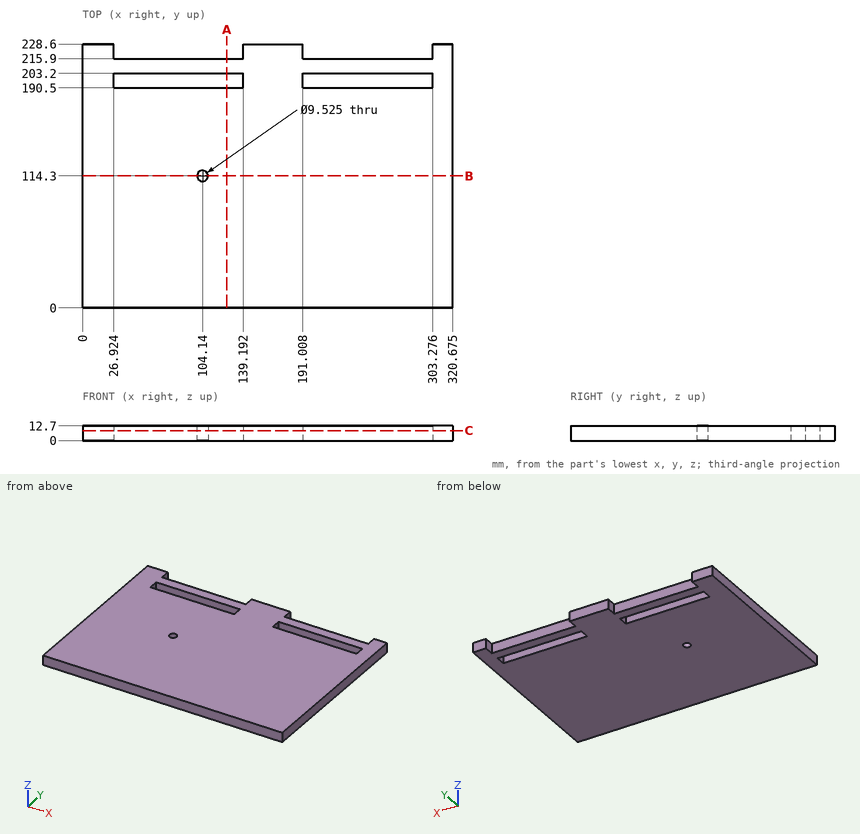
Print and shaded views of the part. All mm, measured from the part's lowest x, y and z. Round coordinates to 2 decimals unless told otherwise and drop trailing zeros. Order: outer loops, then holes, each group sorted by start corner. A loop starts at its lowest first (then second) coordinate and runs counter-clockwise, first axis right, second up.
Q1. Wall check: L1, parallel to X at y = 198, z = 9.75 (3 decimals); L2, parallel to Y at x = 104.14, z = 3.25; L3, parallel to Y at x = 86, z = 11.5. Give the ranges that are in metal, low to high.
Q2. Slice it at B-B (y = 114.3). Write the cut outline in (x, z) (1 decimal).
Q3. Drop a flat-ended pin along its axis: pin 1 (1 mm diameter, centred on x = 260, z = 5, fed in from +Y). Give the stop position or say it passes through.
Q4. Slice it at C-C (z = 8.5). Write the cut outline in (x, y) (1 decimal).
Q5. Slice it at A-A (x = 125). Write the cut outline in (y, z), and give its area (3 significant figures).
Results below:
1. L1: x = 0 to 26.924, 139.192 to 191.008, 303.276 to 320.675
1. L2: y = 0 to 109.54, 119.06 to 190.5, 203.2 to 215.9
1. L3: y = 0 to 190.5, 203.2 to 215.9
2. outline: (0, 0) - (99.4, 0) - (99.4, 12.7) - (0, 12.7) - close; (108.9, 0) - (320.7, 0) - (320.7, 12.7) - (108.9, 12.7) - close
3. pin 1: stops at y = 215.9
4. outline: (0, 0) - (320.7, 0) - (320.7, 228.6) - (303.3, 228.6) - (303.3, 215.9) - (191, 215.9) - (191, 228.6) - (139.2, 228.6) - (139.2, 215.9) - (26.9, 215.9) - (26.9, 228.6) - (0, 228.6) - close; hole (26.9, 190.5) - (139.2, 190.5) - (139.2, 203.2) - (26.9, 203.2) - close; hole circle Ø9.5 at (104.1, 114.3); hole (191, 190.5) - (303.3, 190.5) - (303.3, 203.2) - (191, 203.2) - close
5. outline: (0, 0) - (190.5, 0) - (190.5, 12.7) - (0, 12.7) - close; (203.2, 0) - (215.9, 0) - (215.9, 12.7) - (203.2, 12.7) - close
5. area: 2,580 mm2
